Here's how the part is built. I have some questions about the finished solid (model axes, mm). A direction names the side the tool comes from. Round coordinates to 2 decimals unless told otherwise and drop trailing zeros. Write each loop counter-clockwise with the first axis right and the second up, starting at its lowest first coordinate (ties: lowest second). Pieces come first, ordered by that corner, then holes. Notation, with made-up numbers: (84, 27) -> (102, 27) arc R8 ccw to (102, 39) -> close; hole circle Ø7 at (-25, -16.75). An arc over 180 degrees is marked (long way). Answer as CSV lines item,"result".
from build123d import *

# Parameters (mm, degrees)
SKETCH1_W           = 58.7
SKETCH1_H           = 14.5
BOSS_EXTRUDE1_DEPTH = 2
SKETCH2_W           = 1.907537222
SKETCH2_H           = 8.6
BOSS_EXTRUDE2_DEPTH = 4.3
SKETCH3_W           = 2.3
SKETCH3_H           = 8.6
BOSS_EXTRUDE3_DEPTH = 4.3
FILLET3_R           = 2
SKETCH4_W           = 0.949738238
SKETCH4_H           = 9
BOSS_EXTRUDE4_DEPTH = 12
SKETCH5_W           = 14
SKETCH5_H           = 9.016953004
BOSS_EXTRUDE5_DEPTH = 10
FILLET4_R           = 5.5
CUT_EXTRUDE1_DEPTH  = 12
SKETCH8_W           = 2.580145407
SKETCH8_H           = 9.016953004
SKETCH8_W_2         = 1.5
BOSS_EXTRUDE6_DEPTH = 2
SKETCH9_W           = 1.920869139
SKETCH9_H           = 1.685794619
SKETCH9_H_2         = 1.68579462
BOSS_EXTRUDE7_DEPTH = 3
FILLET6_R           = 3
FILLET9_R           = 3
FILLET11_R          = 1
FILLET12_R          = 1
FILLET13_R          = 2


with BuildPart() as part:
    # Sketch1 → Boss-Extrude1 (new body)
    with BuildSketch(Plane.XY):
        with Locations((15.900667763, -7.24741023)):
            Rectangle(SKETCH1_W, SKETCH1_H)
        with Locations((15.900667763, 7.25258977)):
            Rectangle(SKETCH1_W, SKETCH1_H)
    extrude(amount=BOSS_EXTRUDE1_DEPTH)

    # Sketch2 → Boss-Extrude2 (add)
    with BuildSketch(Plane.XY.offset(2)):
        with Locations((44.296899152, 0)):
            Rectangle(SKETCH2_W, SKETCH2_H)
    extrude(amount=-BOSS_EXTRUDE2_DEPTH)

    # Sketch3 → Boss-Extrude3 (add)
    with BuildSketch(Plane(origin=(45.250667763, 0, 0), x_dir=(0, 0, -1), z_dir=(1, 0, 0))):
        with Locations((1.15, 0)):
            Rectangle(SKETCH3_W, SKETCH3_H)
    extrude(amount=BOSS_EXTRUDE3_DEPTH)

    # Fillet3
    fillet3_edges = [part.edges().sort_by_distance(p)[0] for p in [
        (43.343130541, 0, -2.3),
    ]]
    fillet(fillet3_edges, radius=FILLET3_R)

    # Sketch4 → Boss-Extrude4 (add)
    with BuildSketch(Plane(origin=(0, 0, 0), x_dir=(-1, 0, 0), z_dir=(0, 0, -1))):
        with Locations((12.974463118, 0.00258977)):
            Rectangle(SKETCH4_W, SKETCH4_H)
    extrude(amount=BOSS_EXTRUDE4_DEPTH)

    # Sketch5 → Boss-Extrude5 (add)
    with BuildSketch(Plane.ZY.offset(13.449332237)):
        with Locations((-5, -0.005886732)):
            Rectangle(SKETCH5_W, SKETCH5_H)
    extrude(amount=BOSS_EXTRUDE5_DEPTH)

    # Fillet4
    # the kernel refuses this fillet: 5.5 mm, written as the material it takes off along each edge
    with BuildSketch(Plane(origin=(-23.449332237, -18.264363234, -12), x_dir=(1, 0, 0), z_dir=(0, 1, 0))) as fillet4_piece_1:
        with BuildLine():
            CenterArc((FILLET4_R, -FILLET4_R), FILLET4_R, 90, 90)
            Line((0, -FILLET4_R), (0, 0))
            Line((0, 0), (FILLET4_R, 0))
        make_face()
    extrude(amount=36.516953004, mode=Mode.SUBTRACT)
    with BuildSketch(Plane(origin=(-12.499593999, -18.24741023, -12), x_dir=(-1, 0, 0), z_dir=(0, 1, 0))) as fillet4_piece_2:
        with BuildLine():
            CenterArc((FILLET4_R, FILLET4_R), FILLET4_R, 180, 90)
            Line((0, FILLET4_R), (0, 0))
            Line((0, 0), (FILLET4_R, 0))
        make_face()
    extrude(amount=36.5, mode=Mode.SUBTRACT)

    # Sketch7 → Cut-Extrude1 (cut)
    with BuildSketch(Plane(origin=(0, 4.50258977, 0), x_dir=(1, 0, 0), z_dir=(0, 1, 0))):
        with BuildLine():
            ThreePointArc((-15.03934254, 6.5), (-17.974463118, 9.435120578), (-20.909583696, 6.5))
            Line((-20.909583696, 6.5), (-15.03934254, 6.5))
        make_face()
        with BuildLine():
            Line((-15.03934254, 6.5), (-20.909583696, 6.5))
            ThreePointArc((-20.909583696, 6.5), (-17.974463118, 3.564879422), (-15.03934254, 6.5))
        make_face()
        with BuildLine():
            ThreePointArc((-15.03934254, 6.5), (-17.974463118, 3.564879422), (-20.909583696, 6.5))
            Line((-20.909583696, 6.5), (-20.909583696, -2))
            Line((-20.909583696, -2), (-15.03934254, -2))
            Line((-15.03934254, -2), (-15.03934254, 6.5))
        make_face()
    extrude(amount=-CUT_EXTRUDE1_DEPTH, mode=Mode.SUBTRACT)

    # Sketch8 → Boss-Extrude6 (add)
    with BuildSketch(Plane.ZY.offset(23.449332237)):
        with Locations((-2.790072703, -0.005886732)):
            Rectangle(SKETCH8_W, SKETCH8_H)
        with Locations((1.25, -0.005886732)):
            Rectangle(SKETCH8_W_2, SKETCH8_H)
    extrude(amount=BOSS_EXTRUDE6_DEPTH)

    # Sketch9 → Boss-Extrude7 (add)
    with BuildSketch(Plane(origin=(0, 0, 0), x_dir=(-1, 0, 0), z_dir=(0, 0, -1))):
        with Locations((11.550124457, -3.589191377)):
            Rectangle(SKETCH9_W, SKETCH9_H)
        with Locations((11.539159429, 3.65969246)):
            Rectangle(SKETCH9_W, SKETCH9_H_2)
    extrude(amount=BOSS_EXTRUDE7_DEPTH)

    # Fillet6
    # the kernel refuses this fillet: 3 mm, written as the material it takes off along each edge
    with BuildSketch(Plane(origin=(-10.589689887, 4.241056538, -3), x_dir=(-1, 0, 0), z_dir=(0, -1, 0))) as fillet6_piece_1_section:
        with BuildLine():
            CenterArc((3, -2.794940242), FILLET6_R, 111.307014795, 68.692985205)
            Line((0, -2.794940242), (0, 0))
            Line((0, 0), (1.909904112, 0))
        make_face()
    fillet6_piece_1 = extrude(amount=15.660495829, mode=Mode.PRIVATE)
    fillet6_piece_1 = split(fillet6_piece_1, bisect_by=Plane(origin=(-11.107813793, 2.81679515, -1.901033535), z_dir=(0, -1, 0)), keep=Keep.TOP, mode=Mode.PRIVATE)
    add(fillet6_piece_1, mode=Mode.SUBTRACT)
    with BuildSketch(Plane(origin=(-10.57872486, 11.500570097, -3), x_dir=(-1, 0, 0), z_dir=(0, -1, 0))) as fillet6_piece_2:
        with BuildLine():
            CenterArc((3, -2.799192131), FILLET6_R, 111.082404826, 68.917595174)
            Line((0, -2.799192131), (0, 0))
            Line((0, 0), (1.920869139, 0))
        make_face()
    extrude(amount=15.681755273, mode=Mode.SUBTRACT)

    # Fillet9
    # the kernel refuses this fillet: 3 mm, written as the material it takes off along each edge
    with BuildSketch(Plane(origin=(49.550667763, 11.592976073, -2.3), x_dir=(-1, 0, 0), z_dir=(0, -1, 0))) as fillet9_piece_1:
        with BuildLine():
            CenterArc((2.917190429, -3), FILLET9_R, 90, 76.506601178)
            Line((0, -2.3), (-0.058343809, -2.286))
            ThreePointArc((-0.058343809, -2.286), (-0.06, -1.15), (-0.06, 0))
            Line((-0.06, 0), (0, 0.06))
            Line((0, 0.06), (2.917190429, 0.06))
            Line((2.917190429, 0.06), (2.917190429, 0))
        make_face()
    extrude(amount=23.185952146, mode=Mode.SUBTRACT)

    # Fillet11
    fillet11_edges = [part.edges().sort_by_distance(p)[0] for p in [
        (-25.449332237, -0.005886732, -4.080145407),
        (-25.449332237, -4.514363234, -2.790072704),
        (-25.449332237, -0.005886732, -1.5),
        (-25.449332237, 4.50258977, -2.790072704),
    ]]
    fillet(fillet11_edges, radius=FILLET11_R)

    # Fillet12
    fillet12_edges = [part.edges().sort_by_distance(p)[0] for p in [
        (-25.449332237, 4.50258977, 1.25),
        (-25.449332237, -0.005886732, 0.5),
        (-25.449332237, -4.514363234, 1.25),
    ]]
    fillet(fillet12_edges, radius=FILLET12_R)

    # Fillet13
    fillet13_edges = [part.edges().sort_by_distance(p)[0] for p in [
        (-20.909583696, -0.005886732, 2),
    ]]
    fillet(fillet13_edges, radius=FILLET13_R)


solid = part.part
Item 1: Suppose I cut it at C-C, the plane x = 16. List the corners of the cut face in (y, z) for me.
Results found:
outline,"(-14.5, 0) -> (14.5, 0) -> (14.5, 2) -> (-14.5, 2) -> close"
Item 2: Will these pins go through, and if not, where does the flat tip stop? pin 1 (1.5 mm diameter, centred on x = -12, z = -1.5, fed in from -Y); pin 2 (0.5 mm diameter, centred on x = -24, y = -1, fed in from -Z); pin 3 (2 mm diameter, centred on y = 3, z = -9, fed in from -X); pin 4 (3 mm diameter, centred on x = -11, z = -9, fed in from -Y).
Results found:
pin 1,"stops at y = -4.5"
pin 2,"stops at z = -4.08"
pin 3,"stops at x = -23.24"
pin 4,"passes through"
Item 3: For faces 1 (the cylindrical face through (43.945, 0.06, -1.73)), 2 (the flat face through (-23.449, 0, -1)), 3 (the flat face through (-15.039, 0, -2)), which set-ups out of +Z, -Z, +X, -X, +Y, -Y let a thin tool reach every point of the face, with its end or its side?
Results found:
face 1,"-Z, +Y, -Y"
face 2,"-X, +Y, -Y"
face 3,"+Z, +Y, -Y"
Item 4: I need wall thicknesses on L1, parallel to Z at x = 36.5, y = 7; L2, parallel to X at y = 1.5, z = -2; L3, parallel to X at y = 3.5, z = -9. Which ranges of each line are inside material? Lowest first, please.
Results found:
L1,"z = 0 to 2"
L2,"x = -25.32 to -20.91, -15.04 to -12.5, 44.29 to 47.94"
L3,"x = -22.85 to -19.51, -16.44 to -13.1"
Item 5: Suppose I cut it at A-A, the plane y = 0. List the corners of the cut face in (x, z) for me, then the cut area to 3 significant figures.
Results found:
outline,"(-25.45, -3.08) arc R1 ccw to (-24.45, -4.08) -> (-23.45, -4.08) -> (-23.45, -6.5) arc R5.5 ccw to (-17.97, -12) arc R5.5 ccw to (-12.5, -6.5) -> (-12.5, 0) -> (43.34, 0) -> (43.34, -0.3) arc R2 ccw to (45.34, -2.3) -> (46.63, -2.3) arc R3 ccw to (49.55, 0) -> (45.25, 0) -> (45.25, 2) -> (-15.04, 2) -> (-15.04, -6.5) arc R2.94 cw to (-20.91, -6.5) -> (-20.91, 0) arc R2 ccw to (-22.91, 2) -> (-25.45, 2) -> (-25.45, 1.5) arc R1 ccw to (-24.45, 0.5) -> (-23.45, 0.5) -> (-23.45, -1.5) -> (-24.45, -1.5) arc R1 ccw to (-25.45, -2.5) -> close"
area,"211 mm²"
Item 6: Suppose I cut it at D-D, the plane y = -10.25. List the corners of the cut face in (x, z) for me, then the cut area to 3 significant figures.
Results found:
outline,"(-13.45, 0) -> (45.25, 0) -> (45.25, 2) -> (-13.45, 2) -> close"
area,"117 mm²"
Item 7: If we mould it in two halves opening along Y, with no side actions, what happens to faces 4 (the flat face through (15, -14.497, 1)), 5 (the flat face through (15, 14.503, 1)), 6 (the flat face through (-13.449, 10, 1)), 7 (the flat face through (-12, 2.817, -1))? For each: pulls with the +Y half, pulls with the -Y half, needs draft (parallel to the pull), parting line crosses it, or undercut.
Results found:
face 4,"pulls with the -Y half"
face 5,"pulls with the +Y half"
face 6,"needs draft"
face 7,"undercut"
